Here's how the part is built. I have some questions about the finished solid (model axes, mm). Face numbers are marked on the shaded views. A direction names the side the tool comes from. Coordinates: 2 decimals unless noted, no trailing zeros. Write each loop counter-clockwise with the first axis right and the second up, starting at its lowest first coordinate (ties: lowest second). Pieces come first, ordered by that corner, then holes.
(1) For pin 1 Ø1.8 at (y, z) = (-3, 145) entering from +X; pin 2 Ø0.6 at (x, y) = (23, -2) entering from +Z; pin 3 Ø20 at (x, z) = (3.5, -48.5) entering from +Y, each with a flat end and sliding along its axis, tell me the tip position at first contact or that it passes through.
(2) Imagine slicing it at A-A, the plane x = 4. List the corners of the cut face in (y, z) for me.
(3) Imagine slicing it at D-D, the plane z = 131.5. List the corners of the cut face in (x, y) for me, plus the area to 3 significant figures.
(4) Please list where these lines run through material, in increasing order: probe 1 along Y at (x, z) = (20.5, 80); probe 2 along X at (y, z) = (105, -140); probe 3 along Y at (x, z) = (0, -109.5).
(5) Imagine slicing it at B-B, the plane z = -97.5. List the corners of the cut face in (x, y) for me.
(6) Which directions (+Z, -Z, +X, -X, +Y, -Y) give clear straight access to the entire face, cutting with the end or side of a thin tool? Please do the marked faces 1 and 2.
(7) Imagine slicing it at C-C, the plane y = 73. List the corners of the cut face in (x, z) for me, plus the area to 3 significant figures.
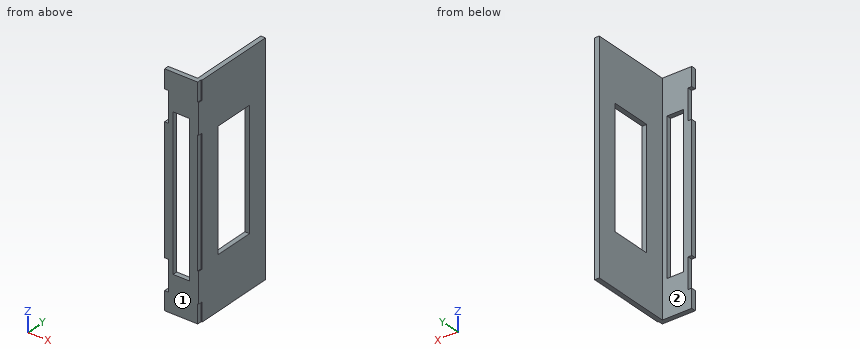
```python
from build123d import *

# Parameters (mm, degrees)
F0_W     = 22.225
F0_H     = 204.7875
F1_DEPTH = 6.35
F3_W     = 55.5625
F3_H     = 161.925
F4_DEPTH = 6.35


with BuildPart() as f1:
    # F0 (on Front) → F1 (new body)
    with BuildSketch(Plane.XZ):
        Polygon((17.4625, 152.4), (-17.4625, 152.4), (-22.5425, 152.4), (-22.5425, 127), (-17.4625, 127), (-17.4625, 85.725), (-22.5425, 85.725), (-22.5425, 0), (-22.5425, -85.725), (-17.4625, -85.725), (-17.4625, -127), (-22.5425, -127), (-22.5425, -152.4), (-17.4625, -152.4), (17.4625, -152.4), (22.5425, -152.4), (22.5425, -127), (17.4625, -127), (17.4625, -85.725), (22.5425, -85.725), (22.5425, 0), (22.5425, 85.725), (17.4625, 85.725), (17.4625, 127), (22.5425, 127), (22.5425, 152.4), align=None)
        Rectangle(F0_W, F0_H, mode=Mode.SUBTRACT)
    extrude(amount=F1_DEPTH)

    # F3 (on offset) → F4 (join)
    with BuildSketch(Plane.YZ.offset(17.4625)):
        Polygon((110.8964, -152.4), (110.8964, 152.4), (-0.2286, 152.4), (-0.2286, 127), (-6.35, 127), (-6.35, 85.725), (-0.2286, 85.725), (-0.2286, -85.725), (-6.35, -85.725), (-6.35, -127), (-0.2286, -127), (-0.2286, -152.4), align=None)
        with Locations((55.3339, 0)):
            Rectangle(F3_W, F3_H, mode=Mode.SUBTRACT)
    extrude(amount=F4_DEPTH)


solid = f1.part
```
Recorded:
1. pin 1: stops at x = 22.54
1. pin 2: stops at z = 127
1. pin 3: stops at y = 0
2. outline: (-6.35, -152.4) - (0, -152.4) - (0, -102.39) - (-6.35, -102.39) - close; (-6.35, 102.39) - (0, 102.39) - (0, 152.4) - (-6.35, 152.4) - close
3. outline: (-22.54, -6.35) - (22.54, -6.35) - (22.54, -0.23) - (23.81, -0.23) - (23.81, 110.9) - (17.46, 110.9) - (17.46, 0) - (-22.54, 0) - close
3. area: 991 mm2
4. probe 1: y = -6.35 to 27.55, 83.12 to 110.9
4. probe 2: x = 17.46 to 23.81
4. probe 3: y = -6.35 to 0
5. outline: (-17.46, -6.35) - (-11.11, -6.35) - (-11.11, 0) - (-17.46, 0) - close; (11.11, -6.35) - (23.81, -6.35) - (23.81, 110.9) - (17.46, 110.9) - (17.46, 0) - (11.11, 0) - close
6. face 1: +Z, -Z, +X, -X, -Y
6. face 2: +Z, -Z, -X, +Y
7. outline: (17.46, -152.4) - (23.81, -152.4) - (23.81, -80.96) - (17.46, -80.96) - close; (17.46, 80.96) - (23.81, 80.96) - (23.81, 152.4) - (17.46, 152.4) - close
7. area: 907 mm2
